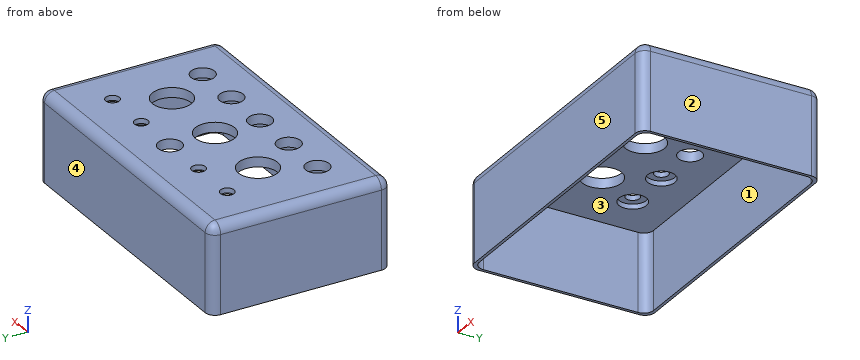
```python
from build123d import *

# Parameters (mm, degrees)
F0_W         = 150
F0_H         = 92
F0_R         = 6
F0_R_2       = 10
F0_R_3       = 3.5
F1_DEPTH     = 2.5
F2_W         = 150
F2_H         = 92
F2_R         = 6
F2_R_2       = 10
F2_R_3       = 7
F3_DEPTH     = 2.5
F4_R         = 4.99999
F5_W         = 150
F5_H         = 92
F6_DEPTH     = 40
F7_T1_DEPTH  = 57.5
F7_T4_ANGLE  = 90
F7_T6_ANGLE  = 90
F7_T8_ANGLE  = 90
F7_T10_ANGLE = 90


# Not quite as in the source:
# - a fillet or chamfer that OpenCascade refuses, or shapes differently, is made with other operations: its cross-section is extruded or revolved along the edge and cut away or added
# - a fillet or chamfer is up to 0.001 mm smaller than in the source, because OpenCascade refuses the exact size


with BuildPart() as f1:
    # F0 (on Top) → F1 (new body)
    with BuildSketch(Plane.XY):
        Rectangle(F0_W, F0_H)
        with Locations((-50, -23)):
            Circle(F0_R, mode=Mode.SUBTRACT)
        with Locations((-25, -23)):
            Circle(F0_R, mode=Mode.SUBTRACT)
        with Locations((0, -23)):
            Circle(F0_R, mode=Mode.SUBTRACT)
        with Locations((25, -23)):
            Circle(F0_R, mode=Mode.SUBTRACT)
        with Locations((50, -23)):
            Circle(F0_R, mode=Mode.SUBTRACT)
        with Locations((-37.5, 0)):
            Circle(F0_R_2, mode=Mode.SUBTRACT)
        with Locations((-50, 23)):
            Circle(F0_R_3, mode=Mode.SUBTRACT)
        with Locations((-25, 23)):
            Circle(F0_R_3, mode=Mode.SUBTRACT)
        Circle(F0_R_2, mode=Mode.SUBTRACT)
        with Locations((37.5, 0)):
            Circle(F0_R_2, mode=Mode.SUBTRACT)
        with Locations((0, 23)):
            Circle(F0_R, mode=Mode.SUBTRACT)
        with Locations((25, 23)):
            Circle(F0_R_3, mode=Mode.SUBTRACT)
        with Locations((50, 23)):
            Circle(F0_R_3, mode=Mode.SUBTRACT)
    extrude(amount=F1_DEPTH)

    # F2 (on Top) → F3 (join)
    with BuildSketch(Plane.XY):
        Rectangle(F2_W, F2_H)
        with Locations((-50, -23)):
            Circle(F2_R, mode=Mode.SUBTRACT)
        with Locations((-25, -23)):
            Circle(F2_R, mode=Mode.SUBTRACT)
        with Locations((0, -23)):
            Circle(F2_R, mode=Mode.SUBTRACT)
        with Locations((25, -23)):
            Circle(F2_R, mode=Mode.SUBTRACT)
        with Locations((50, -23)):
            Circle(F2_R, mode=Mode.SUBTRACT)
        with Locations((-37.5, 0)):
            Circle(F2_R_2, mode=Mode.SUBTRACT)
        with Locations((-50, 23)):
            Circle(F2_R_3, mode=Mode.SUBTRACT)
        with Locations((-25, 23)):
            Circle(F2_R_3, mode=Mode.SUBTRACT)
        Circle(F2_R_2, mode=Mode.SUBTRACT)
        with Locations((37.5, 0)):
            Circle(F2_R_2, mode=Mode.SUBTRACT)
        with Locations((0, 23)):
            Circle(F2_R, mode=Mode.SUBTRACT)
        with Locations((25, 23)):
            Circle(F2_R_3, mode=Mode.SUBTRACT)
        with Locations((50, 23)):
            Circle(F2_R_3, mode=Mode.SUBTRACT)
    extrude(amount=-F3_DEPTH)

    # F4 (radius 5 in the source; OpenCascade refuses exactly that, so slightly less here)
    f4_edges = [f1.edges().sort_by_distance(p)[0] for p in [
        (0, 46, 2.5),
        (-75, 0, 2.5),
        (0, -46, 2.5),
        (75, 0, 2.5),
    ]]
    fillet(f4_edges, radius=F4_R)

    # F5 (on face) → F6 (join)
    with BuildSketch(Plane(origin=(0, 0, -2.5), x_dir=(1, 0, 0), z_dir=(0, 0, -1))):
        Rectangle(F5_W, F5_H)
        with BuildLine():
            ThreePointArc((-73.5, 39.5), (-72.0355339059, 43.0355339059), (-68.5, 44.5))
            Line((-68.5, 44.5), (68.5, 44.5))
            ThreePointArc((68.5, 44.5), (72.0355339059, 43.0355339059), (73.5, 39.5))
            Line((73.5, 39.5), (73.5, -39.5))
            ThreePointArc((73.5, -39.5), (72.0355339059, -43.0355339059), (68.5, -44.5))
            Line((68.5, -44.5), (-68.5, -44.5))
            ThreePointArc((-68.5, -44.5), (-72.0355339059, -43.0355339059), (-73.5, -39.5))
            Line((-73.5, -39.5), (-73.5, 39.5))
        make_face(mode=Mode.SUBTRACT)
    extrude(amount=F6_DEPTH)

    # F7: fillet of radius 5 on 4 edges, made by hand

    # F7_s2 → F7_t1 (cut)
    with BuildSketch(Plane.XY.offset(-55)):
        with BuildLine():
            ThreePointArc((70, -46), (73.5355339059, -44.5355339059), (75, -41))
            Line((75, -41), (75, -46))
            Line((75, -46), (70, -46))
        make_face()
        with BuildLine():
            ThreePointArc((70, 46), (73.5355339059, 44.5355339059), (75, 41))
            Line((75, 41), (75, 46))
            Line((75, 46), (70, 46))
        make_face()
        with BuildLine():
            ThreePointArc((-70, 46), (-73.5355339059, 44.5355339059), (-75, 41))
            Line((-75, 41), (-75, 46))
            Line((-75, 46), (-70, 46))
        make_face()
        with BuildLine():
            ThreePointArc((-70, -46), (-73.5355339059, -44.5355339059), (-75, -41))
            Line((-75, -41), (-75, -46))
            Line((-75, -46), (-70, -46))
        make_face()
    extrude(amount=F7_T1_DEPTH, mode=Mode.SUBTRACT)

    # F7_s3 → F7_t4 (revolve, cut)
    with BuildSketch(Plane.XZ.offset(41)):
        with BuildLine():
            ThreePointArc((-70.00001, 2.5), (-73.5355368349, 1.0355368349), (-75, -2.49999))
            Line((-75, -2.49999), (-75, 2.5))
            Line((-75, 2.5), (-70.00001, 2.5))
        make_face()
    revolve(axis=Axis((-70, -41, 2.5), (0, 0, 1)), revolution_arc=F7_T4_ANGLE, mode=Mode.SUBTRACT)

    # F7_s5 → F7_t6 (revolve, cut)
    with BuildSketch(Plane.YZ.offset(-70)):
        with BuildLine():
            ThreePointArc((41.00001, 2.5), (44.5355368349, 1.0355368349), (46, -2.49999))
            Line((46, -2.49999), (46, 2.5))
            Line((46, 2.5), (41.00001, 2.5))
        make_face()
    revolve(axis=Axis((-70, 41, 2.5), (0, 0, 1)), revolution_arc=F7_T6_ANGLE, mode=Mode.SUBTRACT)

    # F7_s7 → F7_t8 (revolve, cut)
    with BuildSketch(Plane.XZ.offset(-41)):
        with BuildLine():
            ThreePointArc((70.00001, 2.5), (73.5355368349, 1.0355368349), (75, -2.49999))
            Line((75, -2.49999), (75, 2.5))
            Line((75, 2.5), (70.00001, 2.5))
        make_face()
    revolve(axis=Axis((70, 41, 2.5), (0, 0, 1)), revolution_arc=F7_T8_ANGLE, mode=Mode.SUBTRACT)

    # F7_s9 → F7_t10 (revolve, cut)
    with BuildSketch(Plane.YZ.offset(70)):
        with BuildLine():
            ThreePointArc((-41.00001, 2.5), (-44.5355368349, 1.0355368349), (-46, -2.49999))
            Line((-46, -2.49999), (-46, 2.5))
            Line((-46, 2.5), (-41.00001, 2.5))
        make_face()
    revolve(axis=Axis((70, -41, 2.5), (0, 0, 1)), revolution_arc=F7_T10_ANGLE, mode=Mode.SUBTRACT)


solid = f1.part
```
The model under review builds one solid part; all positions refer to its coordinate system, in mm. Face numbers are marked on the shaded views. A direction names the side the tool comes from. Round coordinates to 2 decimals unless told otherwise and drop trailing zeros. Order: outer loops, then holes, each group sorted by start corner. A loop starts at its lowest first (then second) coordinate and runs counter-clockwise, first axis right, second up. Notation, with made-up numbers: (18, -21.75) - (62, -21.75) arc R18 ccw to (62, -2.75) - close; hole circle Ø8 at (75.5, 49.25). An arc over 180 degrees is marked (long way). Answer in a Markdown table with one row per item.
(1) Take a section at A-A on x = -37.5. Write out the cut boundary in (y, z).
Result set:
| item | result |
|---|---|
| outline | (-46, -42.5) - (-44.5, -42.5) - (-44.5, -2.5) - (-10, -2.5) - (-10, 2.5) - (-41, 2.5) arc R5 ccw to (-46, -2.5) - close; (10, -2.5) - (44.5, -2.5) - (44.5, -42.5) - (46, -42.5) - (46, -2.5) arc R5 ccw to (41, 2.5) - (10, 2.5) - close |
(2) Machinability: for the marked faces 1 and 2, which of the approach directions +Z, -Z, +X, -X, +Y, -Y give a long, thin tool a straight path to every point of the face, cutting with its end or side? Answer none if there is none.
Result set:
| item | result |
|---|---|
| face 1 | -Z |
| face 2 | +Z, -Z, +X, +Y, -Y |
(3) Take a section at C-C on z = -18. Write out the cut boundary in (x, y).
Result set:
| item | result |
|---|---|
| outline | (-75, -41) arc R5 ccw to (-70, -46) - (70, -46) arc R5 ccw to (75, -41) - (75, 41) arc R5 ccw to (70, 46) - (-70, 46) arc R5 ccw to (-75, 41) - close; hole (-73.5, -39.5) arc R5 ccw to (-68.5, -44.5) - (68.5, -44.5) arc R5 ccw to (73.5, -39.5) - (73.5, 39.5) arc R5 ccw to (68.5, 44.5) - (-68.5, 44.5) arc R5 ccw to (-73.5, 39.5) - close |
(4) Clearance check with a flat-ended pin moving along its axis: P1, Ø1, axis at x = 20.5, y = 10.5, coming from the -Z side. State where the tip first meets the part, or that it passes through.
Result set:
| item | result |
|---|---|
| P1 | stops at z = -2.5 |
(5) For line 1 (Y direction, x = 45, z = -38); line 2 (X direction, y = 5, z = -7.5); line 3 (Y direction, x = 0, z = 1.45), list the stretches that pass through material, from the lowest coordinate up. Write a range as from..to.
Result set:
| item | result |
|---|---|
| line 1 | y = -46..-44.5, 44.5..46 |
| line 2 | x = -75..-73.5, 73.5..75 |
| line 3 | y = -44.07..-29, -17..-10, 10..17, 29..44.07 |
(6) Take a section at D-D on y = -23. Count the separate pieces of the cut face and the enclosed holes in it, plus the area to 3 significant figures.
Result set:
| item | result |
|---|---|
| separate pieces | 6 |
| enclosed holes | 0 |
| area | 559 mm2 |
(7) Take a section at B-B on y = 0. Write out the cut boundary in (x, z), plus the area to 3 significant figures.
Result set:
| item | result |
|---|---|
| outline | (-75, -42.5) - (-73.5, -42.5) - (-73.5, -2.5) - (-47.5, -2.5) - (-47.5, 2.5) - (-70, 2.5) arc R5 ccw to (-75, -2.5) - close; (-27.5, -2.5) - (-10, -2.5) - (-10, 2.5) - (-27.5, 2.5) - close; (10, -2.5) - (27.5, -2.5) - (27.5, 2.5) - (10, 2.5) - close; (47.5, -2.5) - (73.5, -2.5) - (73.5, -42.5) - (75, -42.5) - (75, -2.5) arc R5 ccw to (70, 2.5) - (47.5, 2.5) - close |
| area | 559 mm2 |
(8) Mouldability with a two-part tool opening along Y and no side actions: class the marked faces 3, 4 and 5 as released by +Y, released by -Y, zero draft, split by the parting line, or undercut.
Result set:
| item | result |
|---|---|
| face 3 | undercut |
| face 4 | released by +Y |
| face 5 | released by -Y |
